Can you work these out from the model? Positions are in its coordinate system, mm. Face numbers are marked on the shaded views. A direction names the side the tool comes from. Round coordinates to 2 decimals unless told otherwise and drop trailing zeros. Loops run counter-clockwise (first coordinate to the right, second up) from the corner with the lowest first, then second, coordinate; pieces in that order, holes last.
from build123d import *

# Parameters (mm, degrees)
F0_W            = 113.76
F0_H            = 69.31
F0_R            = 3
F0_R_2          = 1.5
F1_DEPTH        = 2
F0_W_2          = 118.76
F0_H_2          = 74.31
F2_DEPTH        = 38
F3_W            = 49.53
F3_H            = 23
F4_DEPTH        = 2.5
F5_W            = 16.76
F5_H            = 29
F6_DEPTH        = 2.5
F8_DEPTH        = 2.5
F9_W            = 19.5
F9_H            = 11
F10_DEPTH       = 2
F11_W           = 19.5
F11_H           = 11
F12_DEPTH       = 2
F13_W           = 16.76
F13_H           = 13.5
F14_DEPTH       = 2
F15_W           = 113.76
F15_H           = 33
F16_DEPTH       = 3
F17_W           = 113.76
F17_H           = 1.5
F18_DEPTH       = 2.5
F20_DEPTH       = 1
F22_DEPTH       = 1
F23_D           = 3
F23_DEPTH       = 5
F23_CSINK_D     = 6
F23_CSINK_ANGLE = 90
F23_TIP         = 0.9012909285


with BuildPart() as f1:
    # F0 (on Top) → F1 (new body)
    with BuildSketch(Plane.XY):
        with Locations((55.88, 33.655)):
            Rectangle(F0_W, F0_H)
        with Locations((4.82, 4.82)):
            Circle(F0_R, mode=Mode.SUBTRACT)
        with Locations((106.94, 4.82)):
            Circle(F0_R, mode=Mode.SUBTRACT)
        with Locations((4.82, 62.49)):
            Circle(F0_R, mode=Mode.SUBTRACT)
        with Locations((106.94, 62.49)):
            Circle(F0_R, mode=Mode.SUBTRACT)
        with Locations((106.94, 62.49)):
            Circle(F0_R)
        with Locations((106.94, 62.49)):
            Circle(F0_R_2, mode=Mode.SUBTRACT)
        with Locations((106.94, 62.49)):
            Circle(F0_R_2)
        with Locations((106.94, 4.82)):
            Circle(F0_R)
        with Locations((106.94, 4.82)):
            Circle(F0_R_2, mode=Mode.SUBTRACT)
        with Locations((106.94, 4.82)):
            Circle(F0_R_2)
        with Locations((4.82, 4.82)):
            Circle(F0_R)
        with Locations((4.82, 4.82)):
            Circle(F0_R_2, mode=Mode.SUBTRACT)
        with Locations((4.82, 4.82)):
            Circle(F0_R_2)
        with Locations((4.82, 62.49)):
            Circle(F0_R)
        with Locations((4.82, 62.49)):
            Circle(F0_R_2, mode=Mode.SUBTRACT)
        with Locations((4.82, 62.49)):
            Circle(F0_R_2)
    extrude(amount=F1_DEPTH)

    # F0 (on Top) → F2 (join)
    with BuildSketch(Plane.XY):
        with Locations((55.88, 33.155)):
            Rectangle(F0_W_2, F0_H_2)
        with Locations((55.88, 33.655)):
            Rectangle(F0_W, F0_H, mode=Mode.SUBTRACT)
    extrude(amount=F2_DEPTH)

    # F3 (on face) → F4 (cut, through all)
    with BuildSketch(Plane.YZ.offset(115.26)):
        with Locations((33.655, 20)):
            Rectangle(F3_W, F3_H)
    extrude(amount=-F4_DEPTH, mode=Mode.SUBTRACT)

    # F5 (on face) → F6 (cut, through all)
    with BuildSketch(Plane(origin=(-3.5, 0, 0), x_dir=(0, -1, 0), z_dir=(-1, 0, 0))):
        with Locations((-16, 23.5)):
            Rectangle(F5_W, F5_H)
    extrude(amount=-F6_DEPTH, mode=Mode.SUBTRACT)

    # F7 (on face) → F8 (join)
    with BuildSketch(Plane.XY.offset(38)):
        Polygon((-1, 7.62), (-1, -1), (112.76, -1), (112.76, 68.31), (-1, 68.31), (-1, 24.38), (18.5, 24.38), (18.5, 7.62), align=None)
    extrude(amount=-F8_DEPTH)

    # F9 (on face) → F10 (join)
    with BuildSketch(Plane.XZ.offset(-24.38)):
        with Locations((8.75, 30)):
            Rectangle(F9_W, F9_H)
    extrude(amount=-F10_DEPTH)

    # F11 (on face) → F12 (join)
    with BuildSketch(Plane(origin=(0, 7.62, 0), x_dir=(-1, 0, 0), z_dir=(0, 1, 0))):
        with Locations((-8.75, 30)):
            Rectangle(F11_W, F11_H)
    extrude(amount=-F12_DEPTH)

    # F13 (on face) → F14 (join)
    with BuildSketch(Plane(origin=(18.5, 0, 0), x_dir=(0, -1, 0), z_dir=(-1, 0, 0))):
        with Locations((-16, 31.25)):
            Rectangle(F13_W, F13_H)
    extrude(amount=F14_DEPTH)

    # F15 (on face) → F16 (cut, through all)
    with BuildSketch(Plane.XZ.offset(4)):
        with Locations((55.88, 19)):
            Rectangle(F15_W, F15_H)
    extrude(amount=-F16_DEPTH, mode=Mode.SUBTRACT)

    # F17 (on face) → F18 (cut)
    with BuildSketch(Plane.XZ.offset(4)):
        with Locations((55.88, 36.25)):
            Rectangle(F17_W, F17_H)
        with Locations((55.88, 1.75)):
            Rectangle(F17_W, F17_H)
    extrude(amount=-F18_DEPTH, mode=Mode.SUBTRACT)

    # F19 (on face) → F20 (cut)
    with BuildSketch(Plane.YZ.offset(-1)):
        Polygon((-1.5, 35.5), (-1.5, 37), (-2.5, 37), (-2.5, 1), (-1.5, 1), (-1.5, 2.5), align=None)
    extrude(amount=-F20_DEPTH, mode=Mode.SUBTRACT)

    # F21 (on face) → F22 (cut)
    with BuildSketch(Plane(origin=(112.76, 0, 0), x_dir=(0, -1, 0), z_dir=(-1, 0, 0))):
        Polygon((2.5, 37), (1.5, 37), (1.5, 35.5), (1.5, 2.5), (1.5, 1), (2.5, 1), align=None)
    extrude(amount=-F22_DEPTH, mode=Mode.SUBTRACT)

    # F23
    with Locations(Plane(origin=(0, 0, 0), x_dir=(1, 0, 0), z_dir=(0, 0, -1))):
        with Locations((4.82, -4.82), (106.94, -4.82), (106.94, -62.49), (4.82, -62.49)):
            CounterSinkHole(F23_D / 2, F23_CSINK_D / 2, depth=F23_DEPTH, counter_sink_angle=F23_CSINK_ANGLE)
            with Locations((0, 0, -(F23_DEPTH + F23_TIP / 2))):  # 118° drill point
                Cone(0, F23_D / 2, F23_TIP, mode=Mode.SUBTRACT)


solid = f1.part
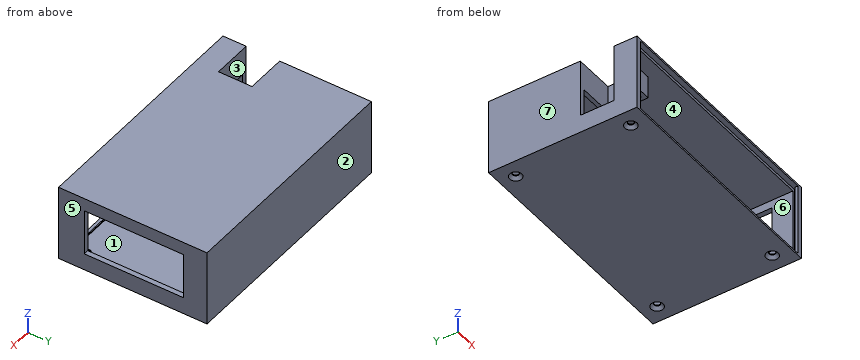
(1) If I drill on line 1 (X direction, y = 62.49, z = 1.7); line 2 (Y direction, x = 4.82, z = 1.8); line 3 (X direction, y = 3, z = 33.5), over which ranges is the centre line in solid material (lowest first)?
Worked answers:
line 1: x = -3.5 to 3.32, 6.32 to 105.44, 108.44 to 115.26
line 2: y = -1.5 to 3.32, 6.32 to 60.99, 63.99 to 70.31
line 3: x = -3.5 to -1, 112.76 to 115.26
(2) If we section it at D-D, the plane y = 31.5: List the corners of the cut face in (x, z) for me.
Worked answers:
outline: (-3.5, 0) - (115.26, 0) - (115.26, 8.5) - (112.76, 8.5) - (112.76, 2) - (-1, 2) - (-1, 35.5) - (112.76, 35.5) - (112.76, 31.5) - (115.26, 31.5) - (115.26, 38) - (-3.5, 38) - close
(3) For the marked faces 1, 2 and 3, which set-ups out of +Z, -Z, +X, -X, +Y, -Y let a thin tool reach every point of the face, with its end or its side?
Worked answers:
face 1: none
face 2: +Z, -Z, +X, -X, +Y
face 3: +Z, -X
(4) If we section it at C-C, the plane z = 19.5: List the corners of the cut face in (x, y) for me, then the cut area to 3 significant figures.
Worked answers:
outline: (-3.5, -4) - (-1, -4) - (-1, -2.5) - (-2, -2.5) - (-2, -1.5) - (-1, -1.5) - (-1, 7.62) - (-3.5, 7.62) - close; (-3.5, 24.38) - (-1, 24.38) - (-1, 68.31) - (112.76, 68.31) - (112.76, 58.42) - (115.26, 58.42) - (115.26, 70.31) - (-3.5, 70.31) - close; (112.76, -4) - (115.26, -4) - (115.26, 8.89) - (112.76, 8.89) - (112.76, -1.5) - (113.76, -1.5) - (113.76, -2.5) - (112.76, -2.5) - close
area: 431 mm2
(5) Will these pins go through, and if not, where does the flat tip stop? P1, Ø17, axis at x = 69, z = 24, coming from the -Y side; P2, Ø3, axis at x = -2, y = 18.5, coming from the +Z side; P3, Ø2.5, axis at x = 106.94, y = 62.49, coming from the -Z side.
Worked answers:
P1: stops at y = 68.31
P2: stops at z = 9
P3: stops at z = 35.5
(6) If we mould it in two halves opening along X, with no side actions, what happens to the marked faces 4, 5, 6 and 7? For each: released by +X, released by -X, zero draft, split by the parting line, or undercut.
Worked answers:
face 4: undercut
face 5: released by +X
face 6: undercut
face 7: released by -X
(7) If we section it at A-A, the plane y = 19: List the corners of the cut face in (x, z) for me.
Worked answers:
outline: (-3.5, 0) - (115.26, 0) - (115.26, 8.5) - (112.76, 8.5) - (112.76, 2) - (-1, 2) - (-1, 9) - (-3.5, 9) - close; (16.5, 24.5) - (18.5, 24.5) - (18.5, 35.5) - (112.76, 35.5) - (112.76, 31.5) - (115.26, 31.5) - (115.26, 38) - (16.5, 38) - close
(8) If we section it at B-B, the plane x = 106.94: List the corners of the cut face in (y, z) for me.
Worked answers:
outline: (-4, 0) - (1.82, 0) - (3.32, 1.5) - (3.32, 2) - (-1, 2) - (-1, 2.5) - (-1.5, 2.5) - (-1.5, 1) - (-4, 1) - close; (-4, 37) - (-1.5, 37) - (-1.5, 35.5) - (68.31, 35.5) - (68.31, 2) - (63.99, 2) - (63.99, 1.5) - (65.49, 0) - (70.31, 0) - (70.31, 38) - (-4, 38) - close; (6.32, 1.5) - (7.82, 0) - (59.49, 0) - (60.99, 1.5) - (60.99, 2) - (6.32, 2) - close
